Design review of the part built by this model. Coordinates are the model's own, in mm. A direction names the side the tool comes from. Give positions to 0.01 mm unless a question says otherwise; leave off trailing zeros. Write each loop counter-clockwise with the first axis right and the second up, starting at its lowest first coordinate (ties: lowest second). Pieces come first, ordered by that corner, then holes. Notation, with made-up numbers: (25.5, 71) -> (48.5, 71) arc R28 cw to (48.5, 97) -> close; hole circle Ø2 at (-36, 12). An arc over 180 degrees is marked (long way). Use CSV: the item, a comma, the result in double quotes.
Autodesk Inventor part; units mm, degrees
ref_plane "YZ Plane" through (0, 0, 0) normal (1, 0, 0) x (0, 1, 0)
ref_plane "XZ Plane" through (0, 0, 0) normal (0, 1, 0) x (-1, 0, 0)
ref_plane "XY Plane" through (0, 0, 0) normal (0, 0, 1) x (1, 0, 0)
sketch "Sketch1" plane through (0, 0, 0) normal (0, 0, 1) x (1, 0, 0)
  line L0 (0, 0) -> (71.842, 71.842)
  line L1 (0, 0) -> (101.6, 0) construction
  line L2 (0, 0) -> (-71.842, 71.842)
  line L3 (0, 0) -> (101.6, 0) construction
  circle A0 centre (-161.6446, 161.6446) radius 133.35
  line L4 (0, 0) -> (101.6, 0)
  arc A1 (-39.7375, 267.2529) -> (-267.2529, 39.7375) centre (-161.6446, 161.6446) ccw
  circle A2 centre (161.6446, -161.6446) radius 133.35
  arc A3 (39.7375, -267.2529) -> (267.2529, -39.7375) centre (161.6446, -161.6446) ccw
  circle A4 centre (-161.6446, -161.6446) radius 133.35
  arc A5 (-267.2529, -39.7375) -> (-39.7375, -267.2529) centre (-161.6446, -161.6446) ccw
  arc A6 (267.2529, 39.7375) -> (39.7375, 267.2529) centre (161.6446, 161.6446) ccw
  circle A7 centre (161.6446, 161.6446) radius 133.35
  spline S0 degree 4 poles (-39.7375, 267.2529) (-20.5214, 245.0712) (0, 181.6818) (20.5214, 245.0712) (39.7375, 267.2529) knots 0 0 0 0 0 1 1 1 1 1
  spline S1 degree 4 poles (-39.7375, -267.2529) (-20.5214, -245.0712) (0, -181.6818) (20.5214, -245.0712) (39.7375, -267.2529) knots 0 0 0 0 0 1 1 1 1 1
  spline S2 degree 4 poles (-267.2529, 39.7375) (-245.0712, 20.5214) (-181.6818, 0) (-245.0712, -20.5214) (-267.2529, -39.7375) knots 0 0 0 0 0 1 1 1 1 1
  spline S3 degree 4 poles (267.2529, 39.7375) (245.0712, 20.5214) (181.6818, 0) (245.0712, -20.5214) (267.2529, -39.7375) knots 0 0 0 0 0 1 1 1 1 1
  line L5 (-161.6446, 161.6446) -> (-161.6446, 89.6025)
  line L6 (-161.6446, 161.6446) -> (-76.5569, 161.6446)
  line L7 (161.6446, -161.6446) -> (161.6446, -113.6338)
  line L8 (161.6446, -161.6446) -> (107.4543, -161.6446)
  arc A8 (56.0363, -39.7375) -> (39.7375, -56.0363) centre (161.6446, -161.6446) ccw
  arc A9 (39.7375, 56.0363) -> (56.0363, 39.7375) centre (161.6446, 161.6446) ccw
  arc A10 (-56.0363, 39.7375) -> (-39.7375, 56.0363) centre (-161.6446, 161.6446) ccw
  arc A11 (-39.7375, -56.0363) -> (-56.0363, -39.7375) centre (-157.2611, -157.2611) ccw
  spline S4 degree 4 poles (-56.0363, 39.7375) (-78.218, 20.5214) (-141.5702, 0.0417) (-78.2738, -20.584) (-56.0363, -39.7375) knots 0 0 0 0 0 1 1 1 1 1
  spline S5 degree 4 poles (-39.7375, -56.0363) (-20.584, -78.2738) (0.0417, -141.5702) (20.5214, -78.218) (39.7375, -56.0363) knots 0 0 0 0 0 1 1 1 1 1
  spline S6 degree 4 poles (-39.7375, 56.0363) (-20.5214, 78.218) (0, 141.6074) (20.5214, 78.218) (39.7375, 56.0363) knots 0 0 0 0 0 1 1 1 1 1
  spline S7 degree 4 poles (56.0363, 39.7375) (78.218, 20.5214) (141.6074, 0) (78.218, -20.5214) (56.0363, -39.7375) knots 0 0 0 0 0 1 1 1 1 1
  point P0 (0, 224.0729)
  point P1 (0, -224.0729)
  point P2 (-224.0729, 0)
  point P3 (224.0729, 0)
  point P4 (-99.2163, 0)
  point P5 (0, -99.2163)
  point P6 (0, 99.2163)
  point P7 (99.2163, 0)
  dimension "d0" = 101.6
  dimension "d1" = 45
  dimension "d2" = 101.6
  dimension "d3" = 135
  dimension "d5" = 228.6
  dimension "d7" = 266.7
  dimension "d9" = 0
  dimension "d14" = 27.94
  dimension "d15" = 0
  dimension "d17" = 0
  dimension "d26" = 43.18
extrude "Extrusion3" add sketch "Sketch1" along normal blind 25.4
properties part number "PropProtector"
(1) Take a section at B-B (y = 120). Write out the cut boundary in (x, z).
Established:
outline,"(-317.47, 0) -> (-288.33, 0) -> (-288.33, 25.4) -> (-317.47, 25.4) -> close; (-34.96, 0) -> (34.96, 0) -> (34.96, 25.4) -> (-34.96, 25.4) -> close; (288.33, 0) -> (317.47, 0) -> (317.47, 25.4) -> (288.33, 25.4) -> close"
(2) For line 1 along X through (y, z) = (163.5, 15.5); line 2 along X through (y, z) = (-110, 10.5); line 3 along Y through (x, z) = (-141, 17.5), list the stretches that pass through material, from the lowest coordinate up. Write a range as [from, to].
Established:
line 1,"x = [-322.92, -294.98], [-28.31, 28.31], [294.98, 322.92]"
line 2,"x = [-314.44, -284.59], [-38.7, 38.7], [284.59, 314.44]"
line 3,"y = [-321.61, -293.39], [-29.9, 29.9], [293.39, 321.61]"
(3) Take a section at A-A (x = -123.5). Write out the cut boundary in (y, z), then the cut area to 3 significant figures.
Established:
outline,"(-318.36, 0) -> (-289.42, 0) -> (-289.42, 25.4) -> (-318.36, 25.4) -> close; (-33.87, 0) -> (33.87, 0) -> (33.87, 25.4) -> (-33.87, 25.4) -> close; (289.42, 0) -> (318.36, 0) -> (318.36, 25.4) -> (289.42, 25.4) -> close"
area,"3,190 mm2"
(4) Mouldability with a two-part tool opening along Y and no side actions: class faces 3 (the face through (288.837, 121.59, 12.522)), 4 (the face through (-49, 49, 0)) as +Y half, -Y half, draft (parallel to the pull), parting line (faces both ways), or undercut.
Established:
face 3,"undercut"
face 4,"draft"
(5) Clearance check with flat-ended pins moving along their axes: pin 1 (2 mm diameter, centred on x = -241, z = 3, fed in from +Y); pin 2 (5 mm diameter, centred on y = 98, z = 4.5, fed in from +X); pin 3 (6 mm diameter, centred on y = 247.5, z = 13.5, fed in from -X). State where each tip first meets the part, or that it passes through.
Established:
pin 1,"stops at y = 302.62"
pin 2,"stops at x = 310.9"
pin 3,"stops at x = -300.03"
(6) Tool access review of faces 1 (the face through (-49, 49, 25.4)), 2 (the face through (-47.48, 47.71, 12.52)): name each direction out of +Z, -Z, +X, -X, +Y, -Y from which nothing blocks a thin tool from reaching the whole face with its end or side.
Established:
face 1,"+Z, +X, -X, +Y, -Y"
face 2,"+Z, -Z"
(7) Take a section at C-C (x = -247.5). State how many separate pieces and enclosed holes the cut face has, then the cut area to 3 significant figures.
Established:
separate pieces,"4"
enclosed holes,"0"
area,"3,450 mm2"
